Autodesk Fusion 360 part; units mm, degrees
sketch "Sketch1" plane through (0, 0, 0) normal (0, 1, 0) x (1, 0, 0)
  circle A0 centre (0, 0) radius 48 construction
  circle A1 centre (0, 0) radius 14 construction
  circle A2 centre (0, 0) radius 9.5 construction
  circle A3 centre (0, 0) radius 8 construction
  line L0 (0, 0) -> (8, 0) construction
  line L1 (0, 0) -> (0, -9.5) construction
  line L2 (0, 0) -> (-8, 0) construction
  line L3 (0, 0) -> (0, 9.5) construction
  circle A4 centre (8, 0) radius 1.5 construction
  circle A5 centre (-8, 0) radius 1.5 construction
  circle A6 centre (0, 9.5) radius 1.5 construction
  circle A7 centre (0, 0) radius 12 construction
  line L4 (8, 0) -> (18, 0) construction
  line L5 (21.1, 0) -> (19.55, 2.6847) construction
  line L6 (19.55, 2.6847) -> (16.45, 2.6847) construction
  line L7 (16.45, 2.6847) -> (14.9, 0) construction
  line L8 (14.9, 0) -> (16.45, -2.6847) construction
  line L9 (16.45, -2.6847) -> (19.55, -2.6847) construction
  line L10 (19.55, -2.6847) -> (21.1, 0) construction
  circle A8 centre (18, 0) radius 3.1 construction
  circle A9 centre (18, 0) radius 1.5
  line L11 (0, 52) -> (-68, 52) construction
  line L12 (-9.7468, 47) -> (-68, 47) construction
  line L13 (-68, 52) -> (-68, 47) construction
  line L14 (-68, 47) -> (-68, 35.633) construction
  line L15 (-68, 35.633) -> (-32.1604, 35.633) construction
  line L16 (-68, 35.633) -> (-68, 30.833) construction
  line L17 (-68, 30.833) -> (-36.7876, 30.833) construction
  line L18 (-68, 30.833) -> (-68, -9.167) construction
  line L19 (-60, -9.167) -> (-47.1165, -9.167)
  line L20 (-68, -9.167) -> (-68, -13.967) construction
  line L21 (-68, -13.967) -> (-45.923, -13.967) construction
  line L22 (-60, -13.967) -> (-60, 35.633)
  line L23 (5.9333, 10.4305) -> (19.5328, 2.6945)
  line L24 (-60, -13.967) -> (21.1, -13.967)
  line L25 (21.1, -13.967) -> (21.1, 0) construction
  arc A10 (21.1, 0) -> (19.5328, 2.6945) centre (18, 0) ccw
  line L26 (-60, 35.633) -> (5, 35.633)
  line L27 (5, 35.633) -> (5, 11.8322)
  arc A11 (5.9333, 10.4305) -> (5.7778, 10.5175) centre (0, 0) ccw
  arc A12 (5, 11.8322) -> (5.7778, 10.5175) centre (6.5, 11.8322) ccw
  arc A13 (5.7778, 10.5175) -> (7.9656, 11.513) centre (6.5, 11.8322) ccw construction
  arc A14 (5.4445, 12.898) -> (5, 11.8322) centre (6.5, 11.8322) ccw construction
  arc A15 (7.9656, 11.513) -> (5.4445, 12.898) centre (6.5, 11.8322) ccw construction
  line L28 (5, 11.8322) -> (5, 10.9087) construction
  arc A16 (5.7778, 10.5175) -> (5, 10.9087) centre (0, 0) ccw construction
  line L29 (-60, 30.833) -> (5, 30.833)
  line L30 (-47.1165, -9.167) -> (21.1, -9.167)
  line L31 (-60, 35.633) -> (-60, 45.633)
  line L32 (-60, 45.633) -> (5, 45.633)
  line L33 (5, 45.633) -> (5, 35.633)
  circle A17 centre (-56, 42) radius 1.5
  circle A18 centre (-40, 42) radius 1.5
  line L34 (-40, 42) -> (0, 0) construction
  circle A19 centre (-55.8448, -4.167) radius 1.5
  line L35 (0, 0) -> (-55.8448, -4.167) construction
  line L36 (-68, -9.167) -> (-60, -9.167) construction
  line L37 (-6, -7.5) -> (7.5, -7.5)
  line L38 (7.5, -7.5) -> (7.5, 7.5)
  line L39 (6, 7.5) -> (-7.5, 7.5)
  line L40 (-7.5, 7.5) -> (-7.5, -7.5)
  line L41 (-7.5, -7.5) -> (7.5, 7.5) construction
  line L42 (-7.5, 7.5) -> (7.5, -7.5) construction
  arc A20 (-7.5, -6) -> (-7.0607, -7.0607) centre (-6, -6) ccw
  arc A21 (-7.0607, -7.0607) -> (-6, -7.5) centre (-6, -6) ccw
  line L43 (-7.5, -7.5) -> (-6, -7.5)
  arc A22 (-6, -7.5) -> (-4.602, -6.5438) centre (-6, -6) ccw construction
  arc A23 (-4.9393, -4.9393) -> (-7.5, -6) centre (-6, -6) ccw construction
  arc A24 (-4.602, -6.5438) -> (-4.9393, -4.9393) centre (-6, -6) ccw construction
  arc A25 (6, -7.5) -> (7.0607, -7.0607) centre (6, -6) ccw
  arc A26 (7.0607, -7.0607) -> (7.5, -6) centre (6, -6) ccw
  arc A27 (7.5, -6) -> (6.5438, -4.602) centre (6, -6) ccw construction
  arc A28 (4.9393, -4.9393) -> (6, -7.5) centre (6, -6) ccw construction
  arc A29 (6.5438, -4.602) -> (4.9393, -4.9393) centre (6, -6) ccw construction
  arc A30 (7.0607, 7.0607) -> (6, 7.5) centre (6, 6) ccw
  arc A31 (7.5, 6) -> (7.0607, 7.0607) centre (6, 6) ccw
  arc A32 (6, 7.5) -> (6.5438, 4.602) centre (6, 6) ccw construction
  arc A33 (7.4916, 5.8417) -> (7.5, 6) centre (6, 6) ccw construction
  arc A34 (6.5438, 4.602) -> (7.4916, 5.8417) centre (6, 6) ccw construction
  arc A35 (-7.0607, 7.0607) -> (-7.5, 6) centre (-6, 6) ccw
  arc A36 (-6.8748, 7.2185) -> (-7.0607, 7.0607) centre (-6, 6) ccw
  arc A37 (-6, 7.5) -> (-6.8748, 7.2185) centre (-6, 6) ccw
  arc A38 (-7.5, 6) -> (-4.8256, 5.0669) centre (-6, 6) ccw construction
  arc A39 (-4.602, 6.5438) -> (-6, 7.5) centre (-6, 6) ccw construction
  arc A40 (-4.8256, 5.0669) -> (-4.602, 6.5438) centre (-6, 6) ccw construction
  line L44 (7.5, 7.5) -> (6, 7.5)
  line L45 (5, 11.8322) -> (5, -13.967) construction
  line L46 (5, -13.967) -> (19.8959, -2.4527)
  line L47 (18, 0) -> (21.1, 0) construction
  line L48 (18, 0) -> (19.8959, -2.4527) construction
  arc A41 (19.8959, -2.4527) -> (21.1, 0) centre (18, 0) ccw
  point P0 (18, 0)
  point P1 (-33.1034, 34.7586)
  point P2 (-47.8669, -3.5717)
  dimension "d1" = 96
  dimension "d2" = 28
  dimension "d3" = 19
  dimension "d4" = 16
  dimension "d5" = 3
  dimension "d6" = 3
  dimension "d7" = 3
  dimension "d8" = 24
  dimension "d9" = 18
  dimension "d10" = 3.1
  dimension "d11" = 60
  dimension "d12" = 3
  dimension "d13" = 52
  dimension "d14" = 68
  dimension "d15" = 68
  dimension "d18" = 5
  dimension "d22" = 16.367
  dimension "d23" = 4.8
  dimension "d24" = 40
  dimension "d25" = 4.8
  dimension "d26" = 8
  dimension "d27" = 3.1
  dimension "d28" = 5
  dimension "d33" = 12
  dimension "d34" = 3
  dimension "d35" = 10
  dimension "d36" = 3
  dimension "d37" = 12
  dimension "d38" = 5
  dimension "d39" = 3
  dimension "d40" = 5
  dimension "d41" = 10
  dimension "d42" = 3
  dimension "d43" = 5
  dimension "d44" = 8
  dimension "d66" = 7.5
  dimension "d67" = 7.5
  dimension "d68" = 15
  dimension "d69" = 15
  dimension "d70" = 3
  dimension "d71" = 3
  dimension "d72" = 3
  dimension "d73" = 3
extrude "Extrude1" add sketch "Sketch1" along normal blind 4.8 contours L19 L22 L23 A10 L27 A11 A12 L29 L30 L46 A41 | L19 L22 L24 L30 L46 | L22 L26 L27 L29 | L26 L31 L32 L33 | L40 A20 A21 L43 | L37 L38 A25 A26 | L39 L40 A35 A36 A37 | L38 A30 A31 L44 makes body 1
fillet "Fillet1" radius 4 2 edges at (5, 2.4, -45.633) (-60, 2.4, -45.633) on bodies 1
sketch "Sketch2" plane through (0, 4.8, 0) normal (0, 1, 0) x (-1, 0, 0)
  arc A0 (56, -45.633) -> (60, -41.633) centre (56, -41.633) ccw
  line L0 (60, -41.633) -> (60, 13.967)
  line L1 (60, 13.967) -> (-5, 13.967)
  arc A1 (-19.8959, 2.4527) -> (-19.5328, -2.6945) centre (-18, 0) ccw
  line L2 (-19.5328, -2.6945) -> (-5.9333, -10.4305)
  arc A2 (-5.9333, -10.4305) -> (-5.7778, -10.5175) centre (0, 0) ccw
  arc A3 (-5, -11.8322) -> (-5.7778, -10.5175) centre (-6.5, -11.8322) ccw
  line L3 (-5, -11.8322) -> (-5, -41.633)
  arc A4 (-5, -41.633) -> (-1, -45.633) centre (-1, -41.633) ccw
  line L4 (-1, -45.633) -> (56, -45.633)
  circle A5 centre (40, -42) radius 1.5
  circle A6 centre (56, -42) radius 1.5
  line L5 (47.1165, 9.167) -> (-21.1, 9.167)
  line L6 (60, 9.167) -> (47.1165, 9.167)
  line L7 (60, -30.833) -> (-5, -30.833)
  line L8 (60, -35.633) -> (-5, -35.633)
  line L9 (-5, 13.967) -> (60, 13.967)
  line L10 (60, 13.967) -> (60, 9.167)
  line L11 (57, 9.167) -> (-5, 9.167)
  line L12 (-5, 9.167) -> (-5, 13.967)
  line L13 (-5, -30.833) -> (57, -30.833)
  line L14 (60, -30.833) -> (60, -35.633)
  line L15 (57, -35.633) -> (-5, -35.633)
  line L16 (-5, -35.633) -> (-5, -30.833)
  line L17 (57, 9.167) -> (60, 8.167)
  line L18 (60, 8.167) -> (60, 9.167)
  line L19 (60, 9.167) -> (57, 9.167) construction
  line L20 (57, -30.833) -> (60, -29.833)
  line L21 (60, -30.833) -> (60, -29.833)
  line L22 (60, -35.633) -> (60, -36.633)
  line L23 (60, -36.633) -> (57, -35.633)
  line L24 (57, -35.633) -> (57, -30.833) construction
  line L25 (57, 9.167) -> (57, -30.833) construction
  line L26 (57, -30.833) -> (60, -30.833) construction
  line L27 (60, -35.633) -> (57, -35.633) construction
  line L28 (-5, 13.967) -> (-19.8959, 2.4527)
  circle A7 centre (-18, 0) radius 1.5
  arc A8 (6, -7.5) -> (7.5, -6) centre (6, -6) ccw
  line L29 (6, -7.5) -> (-6, -7.5)
  arc A9 (-7.5, -6) -> (-6, -7.5) centre (-6, -6) ccw
  line L30 (-7.5, -6) -> (-7.5, 6)
  arc A10 (-6, 7.5) -> (-7.5, 6) centre (-6, 6) ccw
  line L31 (-6, 7.5) -> (6, 7.5)
  arc A11 (7.5, 6) -> (6, 7.5) centre (6, 6) ccw
  line L32 (7.5, 6) -> (7.5, -6)
  circle A12 centre (55.8448, 4.167) radius 1.5
  line L33 (-5, 9.167) -> (-11.2097, 9.167)
  line L34 (-5, 13.967) -> (-11.2097, 9.167)
  dimension "d60" = 3
  dimension "d61" = 1
  dimension "d62" = 1
  dimension "d63" = 1
extrude "Extrude4" cut sketch "Sketch2" against normal blind 1.8 contours L0 L8 L22 L23 | L0 L3 L7 L8 L13 L14 L15 L16 | L0 L7 L20 L21 | L0 L6 L17 L18 | L0 L1 L5 L6 L9 L10 L11 L12 | L5 L12 L28 L33 L34 bodies 1
fillet "Fillet2" radius 3 3 edges at (-57, 3.9, 9.167) (-57, 3.9, -30.833) (-57, 3.9, -35.633) on bodies 1
ref_plane "WorkPlane1" through (-30, 0, 0) normal (1, 0, 0) x (0, 1, 0)
ref_plane "WorkPlane2" through (-25, 0, 0) normal (1, 0, 0) x (0, 1, 0)
split "Split1" by plane through (-30, 0, 0) normal (1, 0, 0) bodies 1 makes body 2 at (-11.8075, 0, -32.9017)
split "Split2" by plane through (-25, 0, 0) normal (1, 0, 0) bodies 2 makes body 3 at (-8.8075, 0, -31.5684)
delete_body "RemoveBody1" bodies 2
move_body "Move1" bodies 3 to x (1, 0, 0) y (0, 1, 0) z (0, 0, 1) at (-5, 0, 0)
combine "Combine1" operation add target body 1 tool bodies 3
Verification items for the finished model (mm, model axes). A direction names the side the tool comes from. Give positions to 0.01 mm unless a question says otherwise; leave off trailing zeros. Order: outer loops, then holes, each group sorted by start corner. A loop starts at its lowest first (then second) coordinate and runs counter-clockwise, first axis right, second up. Notation, with made-up numbers: (39, 75.25) -> (90, 75.25) arc R17 ccw to (90, 101.25) -> close; hole circle Ø3 at (-38, 39). An arc over 180 degrees is marked (long way). Answer as CSV lines item,"result".
Q1. Sectioned sample at D-D on y = 2.1. Count the separate pieces of the cut face and the enclosed holes in it, plus the area to 3 significant figures.
Solutions:
separate pieces,"1"
enclosed holes,"5"
area,"3,540 mm²"
Q2. Release check for a two-part mould opening along X. For faces 6 (the cylindrical face through (-41.2, 2.4, -42.9)), 7 (the cylindrical face through (-58.8, 2.43, -44.49)), 8 (the flat face through (-30, 4.8, -41)), 9 (the flat face through (2.5, 2, 0)) record: +X half, -X half, draft (parallel to the pull), parting line (faces both ways), or undercut.
Solutions:
face 6,"undercut"
face 7,"-X half"
face 8,"draft"
face 9,"undercut"
Q3. Access from +Z, -Z, +X, -X, +Y, -Y to the whole of each face (thin tool, end or side, straight path). Record for faces 1 (the flat face through (7.344, 1.833, 8.29)), 2 (the flat face through (-58.713, 3.913, -30.262)), 3 (the flat face through (-5, 2, -7.5)), 4 (the flat face through (-58.7, 3.9, 8.6)), 5 (the flat face through (-31, 4.8, -11)).
Solutions:
face 1,"+Z, +X, +Y, -Y"
face 2,"-X, +Y"
face 3,"+Y, -Y"
face 4,"+Z, -X, +Y"
face 5,"+Z, -Z, +X, -X, +Y"
Q4. Scan lines: probe 1 along Z at (x, y) = (-56, 1.25); probe 2 along Z at (x, y) = (-8.5, 4.4); probe 3 along X at (y, z) = (3.2, 0). Record each from-to range of solid material in increasing order.
Solutions:
probe 1,"z = -45.63 to -43.5, -40.5 to 2.68, 5.66 to 13.97"
probe 2,"z = -45.63 to -35.63, -30.83 to -7.5, 7.5 to 9.17"
probe 3,"x = -60 to -12.5, 2.5 to 11.5, 14.5 to 16.1"
Q5. Sectioned sample at C-C on x = -23. Record the cut outline in (y, z).
Solutions:
outline,"(0, -45.63) -> (4.8, -45.63) -> (4.8, -35.63) -> (3, -35.63) -> (3, -30.83) -> (4.8, -30.83) -> (4.8, 9.17) -> (3, 9.17) -> (3, 13.97) -> (0, 13.97) -> close"
Q6. Depth check by flat-ended pin: pin 1 (2.5 mm diameter, centred on y = 3.5, z = -29, fed in from +X); pin 2 (1.4 mm diameter, centred on x = -15, y = 4.5, fed in from +Z); pin 3 (1.8 mm diameter, centred on x = -56, z = -42, fed in from -Y); pin 4 (2.5 mm diameter, centred on y = 2, z = 2, fed in from +X). Enter the tip coordinate at first touch or a pass-through.
Solutions:
pin 1,"stops at x = 0"
pin 2,"stops at z = 9.17"
pin 3,"passes through"
pin 4,"stops at x = 16.01"
Q7. Sectioned sample at B-B on z = -4.5. Record the cut outline in (x, y), plus the area to 3 significant figures.
Solutions:
outline,"(-60, 0) -> (-12.5, 0) -> (-12.5, 4.8) -> (-60, 4.8) -> close; (2.5, 0) -> (11.36, 0) -> (11.36, 4.8) -> (2.5, 4.8) -> close"
area,"271 mm²"
Q8. Sectioned sample at A-A on x = -40. Record the cut outline in (y, z), plus the area to 3 significant figures.
Solutions:
outline,"(0, -45.63) -> (4.8, -45.63) -> (4.8, -43.5) -> (0, -43.5) -> close; (0, -40.5) -> (4.8, -40.5) -> (4.8, -35.63) -> (3, -35.63) -> (3, -30.83) -> (4.8, -30.83) -> (4.8, 9.17) -> (3, 9.17) -> (3, 13.97) -> (0, 13.97) -> close"
area,"254 mm²"
